from build123d import *

# Parameters (mm, degrees)
F0_W        = 15
F0_H        = 15
F0_R        = 2.5
F1_DEPTH    = 7
F2_W        = 0.7
F2_H        = 2
F3_DEPTH    = 4.5
F4_T1_DEPTH = 4.5
F5_R        = 5


# Not quite as in the source:
# - a fillet or chamfer that OpenCascade refuses, or shapes differently, is made with other operations: its cross-section is extruded or revolved along the edge and cut away or added


with BuildPart() as f1:
    # F0 (on Top) → F1 (new body)
    with BuildSketch(Plane.XY):
        with Locations((-9.923633188, 7.5)):
            Rectangle(F0_W, F0_H)
        with Locations((-9.923633188, 7.5)):
            Circle(F0_R, mode=Mode.SUBTRACT)
    extrude(amount=F1_DEPTH)

    # F2 (on face) → F3 (join)
    with BuildSketch(Plane.YZ.offset(-2.423633188)):
        Polygon((17, 7.25), (17, 6.5), (19, 6.5), align=None)
        Polygon((17, 6.5), (15, 6.5), (15, 4.5), (15.7, 4.5), (19, 4.5), (19, 6.5), align=None)
        with Locations((15.35, 3.5)):
            Rectangle(F2_W, F2_H)
        Polygon((15.7, 2.5), (15, 2.5), (15, 0.5), (17, 0.5), (19, 0.5), (19, 2.5), align=None)
        Polygon((19, 0.5), (17, 0.5), (17, -0.25), align=None)
    extrude(amount=-F3_DEPTH)

    # F4: fillet of radius 0.5 on 7 edges, made by hand

    # F4_s2 → F4_t1 (join)
    with BuildSketch(Plane.YZ.offset(-6.923633188)):
        with BuildLine():
            ThreePointArc((16.2, 2.5), (15.8464466094, 2.6464466094), (15.7, 3))
            Line((15.7, 3), (15.7, 2.5))
            Line((15.7, 2.5), (16.2, 2.5))
        make_face()
        with BuildLine():
            ThreePointArc((15.7, 4), (15.8464466094, 4.3535533906), (16.2, 4.5))
            Line((16.2, 4.5), (15.7, 4.5))
            Line((15.7, 4.5), (15.7, 4))
        make_face()
        with BuildLine():
            ThreePointArc((16.5, 0.5), (16.8535533906, 0.3535533906), (17, 0))
            Line((17, 0), (17, 0.5))
            Line((17, 0.5), (16.5, 0.5))
        make_face()
        with BuildLine():
            ThreePointArc((16.5, 6.5), (16.8535533906, 6.6464466094), (17, 7))
            Line((17, 7), (17, 6.5))
            Line((17, 6.5), (16.5, 6.5))
        make_face()
        with BuildLine():
            ThreePointArc((15, 7), (15.1464466094, 6.6464466094), (15.5, 6.5))
            Line((15.5, 6.5), (15, 6.5))
            Line((15, 6.5), (15, 7))
        make_face()
        with BuildLine():
            ThreePointArc((15, 0), (15.1464466094, 0.3535533906), (15.5, 0.5))
            Line((15.5, 0.5), (15, 0.5))
            Line((15, 0.5), (15, 0))
        make_face()
    extrude(amount=F4_T1_DEPTH)

    # F5
    f5_edges = [f1.edges().sort_by_distance(p)[0] for p in [
        (-17.423633, 15, 3.5),
        (-17.423633, 0, 3.5),
        (-2.423633, 0, 3.5),
    ]]
    fillet(f5_edges, radius=F5_R)


solid = f1.part
For this review, take the finished solid that the model builds, in its own axes (mm). A direction names the side the tool comes from. Round coordinates to 2 decimals unless told otherwise and drop trailing zeros. Loops run counter-clockwise (first coordinate to the right, second up) from the corner with the lowest first, then second, coordinate; pieces in that order, holes last. Notation, with made-up numbers: (21, 64) - (67, 64) arc R14 ccw to (67, 85) - close; hole circle Ø2 at (18, 65). An arc over 180 degrees is marked (long way). One line per item, written item: value. Start each with the question number.
Item 1: Clearance check with flat-ended pins moving along their axes: pin 1 Ø4.5 at (x, y) = (-9.92, 7.5) entering from +Z; pin 2 Ø7.5 at (x, y) = (-12, 8.5) entering from -Z; pin 3 Ø3 at (x, y) = (-4.5, 18) entering from -Z; pin 4 Ø4 at (x, y) = (-14, 16) entering from +Z. State where each tip first meets the part, or that it passes through.
Item 2: Take a section at C-C (x = -8). Give the boundary of the cut face in (y, z), plus the area to 3 significant figures.
Item 3: Take a section at A-A (z = 1.5). Give the boundary of the cut face in (x, y), plus the area to 3 significant figures.
Item 4: For L1, parallel to Z at x = -10.75, y = 1.25; L2, parallel to X at y = 16.75, z = 5; L3, parallel to Y at x = -8, z = 3, list the stretches that pass through material, from the lowest coordinate up.
Item 5: The part is to be moulded in two halves that separate along Z. For faces 4 (the cylindrical face through (-3.849, 1.504, 3.549)), 5 (the flat face through (-5, 16, 6.5)), 6 (the flat face through (-5, 18, 2.5)), say which applies: +Z half, -Z half, draft (parallel to the pull), parting line (faces both ways), or undercut.
Item 6: For faces 1 (the flat face through (-7, 8, 7)), 2 (the flat face through (-6.924, 15.6, 2.7)), 3 (the flat face through (-5, 16, 0.5)), list the 3-axis set-ups (+Z, -Z, +X, -X, +Y, -Y) from which the entire face can be reached by the end or side of a thin tool; tool diameter is ignored.
Item 7: Take a section at D-D (x = -6.25). Give the boundary of the cut face in (y, z), plus the area to 3 significant figures.
Item 8: Take a section at B-B (y = 7.5). Give the boundary of the cut face in (x, z).
Answer below:
1. pin 1: passes through
1. pin 2: stops at z = 0
1. pin 3: stops at z = -0.25
1. pin 4: stops at z = 7
2. outline: (0, 0) - (5.9, 0) - (5.9, 7) - (0, 7) - close; (9.1, 0) - (15, 0) - (15, 7) - (9.1, 7) - close
2. area: 82.6 mm2
3. outline: (-17.42, 5) arc R5 ccw to (-12.42, 0) - (-7.42, 0) arc R5 ccw to (-2.42, 5) - (-2.42, 19) - (-6.92, 19) - (-6.92, 15) - (-12.42, 15) arc R5 ccw to (-17.42, 10) - close; hole circle Ø5 at (-9.92, 7.5)
3. area: 207 mm2
4. L1: z = 0 to 7
4. L2: x = -6.92 to -2.42
4. L3: y = 0 to 5.9, 9.1 to 15
5. face 4: draft
5. face 5: +Z half
5. face 6: undercut
6. face 1: +Z, +X, -X, -Y
6. face 2: +Z, -Z, -X, +Y
6. face 3: -Z, +X, -X
7. outline: (0.14, 0) - (15, 0) arc R0.5 cw to (15.5, 0.5) - (16.5, 0.5) arc R0.5 cw to (17, 0) - (17, -0.25) - (19, 0.5) - (19, 2.5) - (16.2, 2.5) arc R0.5 cw to (15.7, 3) - (15.7, 4) arc R0.5 cw to (16.2, 4.5) - (19, 4.5) - (19, 6.5) - (17, 7.25) - (17, 7) arc R0.5 cw to (16.5, 6.5) - (15.5, 6.5) arc R0.5 cw to (15, 7) - (0.14, 7) - close
7. area: 123 mm2
8. outline: (-17.42, 0) - (-12.42, 0) - (-12.42, 7) - (-17.42, 7) - close; (-7.42, 0) - (-2.42, 0) - (-2.42, 7) - (-7.42, 7) - close
